```python
from build123d import *

# Parameters (mm, degrees)
F0_R     = 11.3175
F1_DEPTH = 7
F2_SIZE  = 1


with BuildPart() as f1:
    # F0 (on Top) → F1 (new body)
    with BuildSketch(Plane.XY):
        with BuildLine():
            ThreePointArc((7.3127307082, -13.0967159849), (12.9362081118, -7.5930573347), (15, 0))
            ThreePointArc((15, 0), (14.9996135208, 0.1076764883), (14.9984541032, 0.2153474281))
            ThreePointArc((14.9984541032, 0.2153474281), (12.9903810568, 7.5), (7.6857233949, 12.8813685568))
            ThreePointArc((7.6857233949, 12.8813685568), (0, 15), (-7.6857233949, 12.8813685568))
            ThreePointArc((-7.6857233949, 12.8813685568), (-12.9903810568, 7.5), (-14.9984541032, 0.2153474281))
            ThreePointArc((-14.9984541032, 0.2153474281), (-12.9903810568, -7.5), (-7.3127307082, -13.0967159849))
            ThreePointArc((-7.3127307082, -13.0967159849), (0, -15), (7.3127307082, -13.0967159849))
        make_face()
        Circle(F0_R, mode=Mode.SUBTRACT)
        with BuildLine():
            ThreePointArc((14.9984541032, 0.2153474281), (14.9996135208, 0.1076764883), (15, 0))
            ThreePointArc((15, 0), (12.9362081118, -7.5930573347), (7.3127307082, -13.0967159849))
            Line((7.3127307082, -13.0967159849), (19.70522071, -34.2219280102))
            ThreePointArc((19.70522071, -34.2219280102), (37.513895389, -21.6586576012), (39.4896693783, 0.0457422831))
            Line((39.4896693783, 0.0457422831), (14.9984541032, 0.2153474281))
        make_face()
        with Locations((25.0325276728, -14.4525365904)):
            Circle(F0_R, mode=Mode.SUBTRACT)
        with BuildLine():
            ThreePointArc((-7.6857233949, 12.8813685568), (0, 15), (7.6857233949, 12.8813685568))
            Line((7.6857233949, 12.8813685568), (19.7844486684, 34.1761857271))
            ThreePointArc((19.7844486684, 34.1761857271), (0, 43.3173152024), (-19.7844486684, 34.1761857271))
            Line((-19.7844486684, 34.1761857271), (-7.6857233949, 12.8813685568))
        make_face()
        with Locations((0, 28.9050731808)):
            Circle(F0_R, mode=Mode.SUBTRACT)
        with BuildLine():
            Line((-19.70522071, -34.2219280102), (-7.3127307082, -13.0967159849))
            ThreePointArc((-7.3127307082, -13.0967159849), (-12.9903810568, -7.5), (-14.9984541032, 0.2153474281))
            Line((-14.9984541032, 0.2153474281), (-39.4896693783, 0.0457422831))
            ThreePointArc((-39.4896693783, 0.0457422831), (-37.513895389, -21.6586576012), (-19.70522071, -34.2219280102))
        make_face()
        with Locations((-25.0325276728, -14.4525365904)):
            Circle(F0_R, mode=Mode.SUBTRACT)
    extrude(amount=F1_DEPTH)

    # F2
    f2_edges = [f1.edges().sort_by_distance(p)[0] for p in [
        (-27.244062, 0.130545, 7),
        (-13.735086, 23.528777, 7),
        (27.244062, 0.130545, 7),
        (13.735086, 23.528777, 7),
        (13.508976, -23.659322, 7),
        (-13.508976, -23.659322, 7),
        (-37.513895, -21.658658, 7),
        (37.513895, -21.658658, 7),
        (0, 43.317315, 7),
        (-12.990381, 7.5, 7),
        (12.990381, 7.5, 7),
        (0, -15, 7),
        (0, -15, 0),
        (13.508976, -23.659322, 0),
        (-13.508976, -23.659322, 0),
        (37.513895, -21.658658, 0),
        (27.244062, 0.130545, 0),
        (12.990381, 7.5, 0),
        (13.735086, 23.528777, 0),
        (0, 43.317315, 0),
        (-13.735086, 23.528777, 0),
        (-12.990381, 7.5, 0),
        (-27.244062, 0.130545, 0),
        (-37.513895, -21.658658, 0),
    ]]
    chamfer(f2_edges, length=F2_SIZE)


solid = f1.part
```
Check sheet for the modelled part. Datum: model origin and axes. Units: mm. A direction names the side the tool comes from. Coordinates: 2 decimals unless noted, no trailing zeros. Write each loop counter-clockwise with the first axis right and the second up, starting at its lowest first coordinate (ties: lowest second). Pieces come first, ordered by that corner, then holes. Notation, with made-up numbers: M 40,39.5 L 95,39.5 A33 ccw 95,72.5 Z; hole C 44,1 d10. An arc over 180 degrees is marked long. Write item = value, one per line. Start each with the question number.
1. Sectioned sample at A-A (x = 0). Record the cut outline in (y, z).
2. Thickness scan on probe 1 along Y at (x, z) = (0, 4); probe 2 along X at (y, z) = (-12, 3.75); probe 3 along Y at (x, z) = (2, 4.5). Record the ranges inside material, lowest first.
3. Sectioned sample at C-C (y = -16.5). State how many separate pieces and enclosed holes the cut face has, then the cut area to 3 significant figures.
4. Go/stop test with flat-tipped pins: pin 1 (1.5 mm diameter, centred on x = 6, z = 5.5, fed in from -Y); pin 2 (3 mm diameter, centred on y = -22.5, z = 5.5, fed in from +X); pin 3 (4 mm diameter, centred on y = 18, z = 2, fed in from +X). Record where each tip stops, or that it passes through.
5. Mould release check, pull along Y, two halves, no side actions. Record for faces 4 (the flat face through (-13.78, -23.12, 6.507)), 5 (the cylindrical face through (5.222, 18.865, 3.451)), 6 (the cylindrical face through (-37.67, -21.385, 3.465)): pulls with the +Y half, pulls with the -Y half, needs draft (parallel to the pull), parting line crosses it, or undercut.
6. Sectioned sample at B-B (z = 4.5). Record the cut outline in (x, y) (1 decimal).
7. Tool access check on faces 1 (the flat face through (13.42, -23.51, 3.47)), 2 (the flat face through (13.65, 23.38, 3.46)), 3 (the cylindrical face through (-12.94, 7.59, 3.47)). Record the directions out of +Z, -Z, +X, -X, +Y, -Y that give a thin tool (end or side, any length) a straight path to the whole face; none if there is none.
The answers:
q1.outline = M -15,1 L -14,0 L -11.32,0 L -11.32,7 L -14,7 L -15,6 Z; M 11.32,0 L 17.59,0 L 17.59,7 L 11.32,7 Z; M 40.22,0 L 42.32,0 L 43.32,1 L 43.32,6 L 42.32,7 L 40.22,7 Z
q2.probe_1 = -15 to -11.32, 11.32 to 17.59, 40.22 to 43.32
q2.probe_2 = -40.78 to -36.08, -13.98 to 13.98, 36.08 to 40.78
q2.probe_3 = -14.87 to -11.14, 11.14 to 17.77, 40.04 to 43.24
q3.separate_pieces = 4
q3.enclosed_holes = 0
q3.area = 111 mm²
q4.pin_1 = -14.05
q4.pin_2 = 37.88
q4.pin_3 = 11.73
q5.face_4 = pulls with the -Y half
q5.face_5 = undercut
q5.face_6 = parting line crosses it
q6.outline = M -39.5,0 A26 ccw -19.7,-34.2 L -7.3,-13.1 A15 ccw 7.3,-13.1 L 19.7,-34.2 A26 ccw 39.5,0 L 15,0.2 A15 ccw 7.7,12.9 L 19.8,34.2 A26 ccw -19.8,34.2 L -7.7,12.9 A15 ccw -15,0.2 Z; hole C -25,-14.5 d22.6; hole C 0,0 d22.6; hole C 0,28.9 d22.6; hole C 25,-14.5 d22.6
q7.face_1 = +Z, -Z, -Y
q7.face_2 = +Z, -Z, +X
q7.face_3 = +Z, -Z, -X
